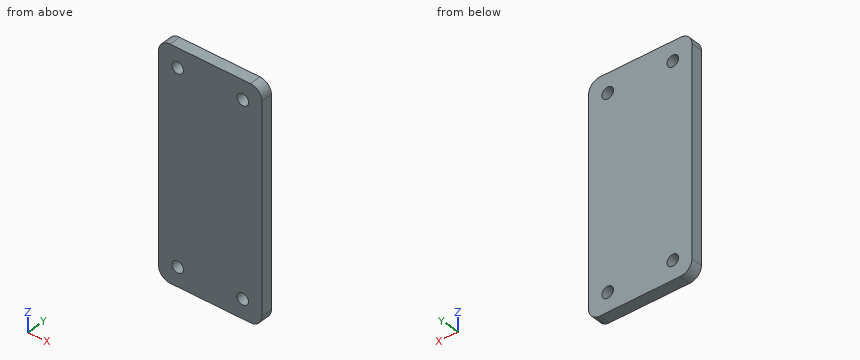
```python
from build123d import *

# Parameters (mm, degrees)
SKETCH3_W           = 27
SKETCH3_H           = 60
BOSS_EXTRUDE1_DEPTH = 3
SKETCH4_R           = 1.5
CUT_EXTRUDE1_DEPTH  = 3
FILLET2_R           = 3
FILLET3_R           = 3


with BuildPart() as part:
    # Sketch3 → Boss-Extrude1 (new body)
    with BuildSketch(Plane(origin=(0, 0, 0), x_dir=(1, 0, 0), z_dir=(0, 1, 0))):
        Rectangle(SKETCH3_W, SKETCH3_H)
    extrude(amount=BOSS_EXTRUDE1_DEPTH)

    # Sketch4 → Cut-Extrude1 (cut)
    with BuildSketch(Plane(origin=(0, 3, 0), x_dir=(1, 0, 0), z_dir=(0, 1, 0))):
        with Locations((-8.5, 25)):
            Circle(SKETCH4_R)
        with Locations((8.5, 25)):
            Circle(SKETCH4_R)
        with Locations((8.5, -25)):
            Circle(SKETCH4_R)
        with Locations((-8.5, -25)):
            Circle(SKETCH4_R)
    extrude(amount=-CUT_EXTRUDE1_DEPTH, mode=Mode.SUBTRACT)

    # Fillet2
    fillet2_edges = [part.edges().sort_by_distance(p)[0] for p in [
        (-13.5, 1.5, 30),
    ]]
    fillet(fillet2_edges, radius=FILLET2_R)

    # Fillet3
    fillet3_edges = [part.edges().sort_by_distance(p)[0] for p in [
        (-13.5, 1.5, -30),
        (13.5, 1.5, -30),
        (13.5, 1.5, 30),
    ]]
    fillet(fillet3_edges, radius=FILLET3_R)


solid = part.part
```
Work out the finished part from the listing and answer in its coordinate system (mm). Round coordinates to 2 decimals unless told otherwise and drop trailing zeros. Order: outer loops, then holes, each group sorted by start corner. A loop starts at its lowest first (then second) coordinate and runs counter-clockwise, first axis right, second up.
Q1. Find the intervals of material crossed by line 1 along Z through (x, y) = (8.5, 2.05); line 2 along X through (y, z) = (2, 25); line 3 along X through (y, z) = (2.3, -25.5), in increasing order.
Solution:
line 1: z = -30 to -26.5, -23.5 to 23.5, 26.5 to 30
line 2: x = -13.5 to -10, -7 to 7, 10 to 13.5
line 3: x = -13.5 to -9.91, -7.09 to 7.09, 9.91 to 13.5
Q2. A cutting plane is placed at A-A, the plane z = 25. Determine the outline of the cut face in (x, y), then the cut area to 3 significant figures.
Solution:
outline: (-13.5, 0) - (-10, 0) - (-10, 3) - (-13.5, 3) - close; (-7, 0) - (7, 0) - (7, 3) - (-7, 3) - close; (10, 0) - (13.5, 0) - (13.5, 3) - (10, 3) - close
area: 63.0 mm2
Q3. A cutting plane is placed at B-B, the plane y = 2.3. Determine the outline of the cut face in (x, z), then the cut area to 3 significant figures.
Solution:
outline: (-13.5, -27) arc R3 ccw to (-10.5, -30) - (10.5, -30) arc R3 ccw to (13.5, -27) - (13.5, 27) arc R3 ccw to (10.5, 30) - (-10.5, 30) arc R3 ccw to (-13.5, 27) - close; hole circle Ø3 at (-8.5, -25); hole circle Ø3 at (-8.5, 25); hole circle Ø3 at (8.5, -25); hole circle Ø3 at (8.5, 25)
area: 1,580 mm2
Q4. A cutting plane is placed at C-C, the plane x = 8.5. Determine the outline of the cut face in (y, z).
Solution:
outline: (0, -30) - (3, -30) - (3, -26.5) - (0, -26.5) - close; (0, -23.5) - (3, -23.5) - (3, 23.5) - (0, 23.5) - close; (0, 26.5) - (3, 26.5) - (3, 30) - (0, 30) - close
